```python
from build123d import *

# Parameters (mm, degrees)
F0_R           = 50.8
F1_DEPTH       = 127
F3_D           = 0.0254
F3_DEPTH       = 123.825
F3_CBORE_D     = 97.79
F3_CBORE_DEPTH = 123.825
F3_TIP         = 0.0076309299
F4_R           = 0.79375


with BuildPart() as f1:
    # F0 (on Top) → F1 (new body)
    with BuildSketch(Plane.XY):
        Circle(F0_R)
    extrude(amount=-F1_DEPTH)

    # F3
    with Locations(Plane.XY):
        with Locations((0, 0)):
            CounterBoreHole(F3_D / 2, F3_CBORE_D / 2, F3_CBORE_DEPTH, depth=F3_DEPTH)
            with Locations((0, 0, -(F3_DEPTH + F3_TIP / 2))):  # 118° drill point
                Cone(0, F3_D / 2, F3_TIP, mode=Mode.SUBTRACT)

    # F4
    f4_edges = [f1.edges().sort_by_distance(p)[0] for p in [
        (-50.8, 0, 0),
        (-48.895, 0, 0),
    ]]
    fillet(f4_edges, radius=F4_R)


solid = f1.part
```
Check sheet for the modelled part. Datum: model origin and axes. Units: mm. Coordinates: 2 decimals unless noted, no trailing zeros. Loops run counter-clockwise (first coordinate to the right, second up) from the corner with the lowest first, then second, coordinate; pieces in that order, holes last. Notation, with made-up numbers: M 74.25,81.25 L 87.25,81.25 A30 ccw 87.25,108.25 Z; hole C -11.75,6 d10. An arc over 180 degrees is marked long. Answer as a JSON object with one key per item and string values.
1. Release check for a two-part mould opening along X. For faces 1 (the flat face through (-1, 1, -123.825)), 2 (the flat face through (-1, 1, -127)), 3 (the cylindrical face through (-11.012, -49.592, -63.013)) record: pulls with the +X half, pulls with the -X half, needs draft (parallel to the pull), parting line crosses it, or undercut.
Outcome:
{"face 1": "undercut", "face 2": "needs draft", "face 3": "parting line crosses it"}
2. Sectioned sample at A-A on z = -101. Record the cut outline in (x, y) (3 decimals).
Outcome:
{"outline": "C 0,0 d101.6; hole C 0,0 d97.79"}
3. Scan lines: L1, parallel to Y at x = 0, z = -31 (3 decimals); L2, parallel to X at y = -10, z = -110.5; L3, parallel to Z at x = -2, y = -33.5 (3 decimals). Record each from-to range of solid material in increasing order. Write a range as from..to.
Outcome:
{"L1": "-50.8..-48.895, 48.895..50.8", "L2": "-49.81..-47.86, 47.86..49.81", "L3": "-127..-123.825"}
4. Depth check by flat-ended pin: P1, Ø4, axis at x = -24, z = -104, coming from the +Y side; P2, Ø2, axis at x = 18, z = -36.5, coming from the -Y side; P3, Ø2, axis at y = -28, z = -84.5, coming from the +X side. Enter the tip coordinate at first touch or a pass-through.
Outcome:
{"P1": "y = 45.79", "P2": "y = -47.87", "P3": "x = 43.03"}
